Design review of the part built by this model. Coordinates are the model's own, in mm. A direction names the side the tool comes from. Coordinates: 2 decimals unless noted, no trailing zeros. Write each loop counter-clockwise with the first axis right and the second up, starting at its lowest first coordinate (ties: lowest second). Pieces come first, ordered by that corner, then holes. Notation, with made-up numbers: (-5.5, 13.5) -> (35.5, 13.5) arc R19 ccw to (35.5, 45.5) -> close; hole circle Ø7 at (31.5, 74). An arc over 180 degrees is marked (long way). Write item = value, one per line. Start each with the question number.
```python
from build123d import *

# Parameters (mm, degrees)
BOSS_EXTRUDE1_DEPTH      = 90
BOSS_EXTRUDE1_DEPTH_BACK = 10
SKETCH1_W                = 120
SKETCH1_H                = 100
FILLET1_R                = 10
SKETCH2_W                = 80
SKETCH2_H                = 60
CUT_EXTRUDE1_DEPTH       = 127.885775404
SKETCH3_W                = 106.2
SKETCH3_H                = 86.2
SKETCH3_W_2              = 93.8
SKETCH3_H_2              = 73.8
CUT_EXTRUDE2_DEPTH       = 10
BOSS_EXTRUDE3_START      = -20
BOSS_EXTRUDE3_DEPTH      = 80
CUT_EXTRUDE3_START       = -30
SKETCH5_R                = 1.25
CUT_EXTRUDE3_DEPTH       = 60
CUT_EXTRUDE4_DEPTH       = 2.5
SKETCH7_W                = 60
SKETCH7_H                = 4
CUT_EXTRUDE5_DEPTH       = 6
FILLET2_R                = 1.5


with BuildPart() as part:
    # Sketch1 → Boss-Extrude1 (new, two sides: drawn at the far end of the back side and taken through both)
    with BuildSketch(Plane(origin=(0, 0, 0), x_dir=(1, 0, 0), z_dir=(0, 1, 0)).offset(-BOSS_EXTRUDE1_DEPTH_BACK)):
        Rectangle(SKETCH1_W, SKETCH1_H)
    extrude(amount=BOSS_EXTRUDE1_DEPTH + BOSS_EXTRUDE1_DEPTH_BACK)

    # Fillet1
    fillet1_edges = [part.edges().sort_by_distance(p)[0] for p in [
        (-60, 40, -50),
        (60, 40, -50),
        (60, 40, 50),
        (-60, 40, 50),
    ]]
    fillet(fillet1_edges, radius=FILLET1_R)

    # Sketch2 → Cut-Extrude1 (cut, through all)
    with BuildSketch(Plane(origin=(0, 90, 0), x_dir=(1, 0, 0), z_dir=(0, 1, 0))):
        Rectangle(SKETCH2_W, SKETCH2_H)
    extrude(amount=-CUT_EXTRUDE1_DEPTH, mode=Mode.SUBTRACT)

    # Sketch3 → Cut-Extrude2 (cut)
    with BuildSketch(Plane.XZ.offset(10)):
        Rectangle(SKETCH3_W, SKETCH3_H)
        Rectangle(SKETCH3_W_2, SKETCH3_H_2, mode=Mode.SUBTRACT)
    extrude(amount=-CUT_EXTRUDE2_DEPTH, mode=Mode.SUBTRACT)

    # Sketch4 → Boss-Extrude3 (add)
    with BuildSketch(Plane(origin=(60, 0, 0), x_dir=(0, 0, -1), z_dir=(1, 0, 0)).offset(BOSS_EXTRUDE3_START)):
        with BuildLine():
            Line((30, 80), (30, 90))
            ThreePointArc((30, 90), (25, 85), (30, 80))
        make_face()
    extrude(amount=-BOSS_EXTRUDE3_DEPTH)

    # Sketch5 → Cut-Extrude3 (cut)
    with BuildSketch(Plane(origin=(60, 0, 0), x_dir=(0, 0, -1), z_dir=(1, 0, 0)).offset(CUT_EXTRUDE3_START)):
        with BuildLine():
            Line((30, 80), (30, 90))
            ThreePointArc((30, 90), (25, 85), (30, 80))
        make_face()
        with Locations((27.5, 85)):
            Circle(SKETCH5_R, mode=Mode.SUBTRACT)
    extrude(amount=-CUT_EXTRUDE3_DEPTH, mode=Mode.SUBTRACT)

    # Sketch6 → Cut-Extrude4 (cut)
    with BuildSketch(Plane(origin=(0, 90, 0), x_dir=(1, 0, 0), z_dir=(0, 1, 0))):
        with BuildLine():
            Line((-40, -30), (-40, 24))
            Line((-40, 24), (-42, 24))
            Line((-42, 24), (-42, -32))
            Line((-42, -32), (-10.392304845, -32))
            ThreePointArc((-10.392304845, -32), (0, -38), (10.392304845, -32))
            Line((10.392304845, -32), (42, -32))
            Line((42, -32), (42, 24))
            Line((42, 24), (40, 24))
            Line((40, 24), (40, -30))
            Line((40, -30), (-40, -30))
        make_face()
    extrude(amount=-CUT_EXTRUDE4_DEPTH, mode=Mode.SUBTRACT)

    # Sketch7 → Cut-Extrude5 (cut)
    with BuildSketch(Plane(origin=(0, 90, 0), x_dir=(1, 0, 0), z_dir=(0, 1, 0))):
        with Locations((0, 32)):
            Rectangle(SKETCH7_W, SKETCH7_H)
    extrude(amount=-CUT_EXTRUDE5_DEPTH, mode=Mode.SUBTRACT)

    # Fillet2
    fillet2_edges = [part.edges().sort_by_distance(p)[0] for p in [
        (-42, 90, 4),
        (-26.196152423, 90, 32),
        (0, 90, 38),
        (26.196152423, 90, 32),
        (42, 90, 4),
        (0, 84, -34),
        (0, 84, -30),
        (0, 90, -34),
    ]]
    fillet(fillet2_edges, radius=FILLET2_R)


solid = part.part
```
(1) For line 1 (Z direction, x = 37.5, y = 69.5); line 2 (X direction, y = 39, z = 18); line 3 (Y direction, x = 52, z = 32), list the stretches that pass through material, from the lowest coordinate up.
(2) Take a section at A-A, the plane z = 16. State the section outline as (x, y) points.
(3) For pin 1 Ø10 at (x, z) = (-31.5, -4) entering from -Y, flat-tipped, find the tip position at first contact; note if it passes through.
(4) Take a section at D-D, the plane y = 44. State the section outline as (x, z) points.
(5) Take a section at C-C, the plane x = 13.5. State the section outline as (y, z) points, then the cut area to 3 significant figures.
(6) Take a section at B-B, the plane x = 32.5. State the section outline as (y, z) points, then the cut area to 3 significant figures.
(7) For faces 1 (the face through (-35, 85, -25)), 2 (the face through (-1, -5, -43.1)), 3 (the face through (0, 87, -34)), 4 (the face through (-1, 39, 30)), 5 (the face through (-60, 39, 1)), list the 3-axis set-ups (+Z, -Z, +X, -X, +Y, -Y) from which the entire face can be reached by the end or side of a thin tool; tool diameter is ignored.
Report:
q1.line_1 = -50 to -30, 30 to 50
q1.line_2 = -60 to -40, 40 to 60
q1.line_3 = 0 to 90
q2.outline = (-60, -10) -> (-53.1, -10) -> (-53.1, 0) -> (-46.9, 0) -> (-46.9, -10) -> (-40, -10) -> (-40, 87.5) -> (-42, 87.5) -> (-42, 88.5) arc R1.5 ccw to (-43.5, 90) -> (-60, 90) -> close; (40, -10) -> (46.9, -10) -> (46.9, 0) -> (53.1, 0) -> (53.1, -10) -> (60, -10) -> (60, 90) -> (43.5, 90) arc R1.5 ccw to (42, 88.5) -> (42, 87.5) -> (40, 87.5) -> close
q3.pin_1 = through
q4.outline = (-60, -40) arc R10 ccw to (-50, -50) -> (50, -50) arc R10 ccw to (60, -40) -> (60, 40) arc R10 ccw to (50, 50) -> (-50, 50) arc R10 ccw to (-60, 40) -> close; hole (-40, -30) -> (40, -30) -> (40, 30) -> (-40, 30) -> close
q5.outline = (-10, -50) -> (90, -50) -> (90, -35.5) arc R1.5 ccw to (88.5, -34) -> (85.5, -34) arc R1.5 cw to (84, -32.5) -> (84, -31.5) arc R1.5 ccw to (82.5, -30) -> (-10, -30) -> (-10, -36.9) -> (0, -36.9) -> (0, -43.1) -> (-10, -43.1) -> close; (-10, 30) -> (87.5, 30) -> (87.5, 32) -> (88.5, 32) arc R1.5 ccw to (90, 33.5) -> (90, 50) -> (-10, 50) -> (-10, 43.1) -> (0, 43.1) -> (0, 36.9) -> (-10, 36.9) -> close; circle Ø2.5 at (85, -27.5)
q5.area = 3,850 mm2
q6.outline = (-10, -50) -> (90, -50) -> (90, -30) arc R5 ccw to (80, -30) -> (-10, -30) -> (-10, -36.9) -> (0, -36.9) -> (0, -43.1) -> (-10, -43.1) -> close; (-10, 30) -> (87.5, 30) -> (87.5, 32) -> (88.5, 32) arc R1.5 ccw to (90, 33.5) -> (90, 50) -> (-10, 50) -> (-10, 43.1) -> (0, 43.1) -> (0, 36.9) -> (-10, 36.9) -> close
q6.area = 3,910 mm2
q7.face_1 = none
q7.face_2 = -Y
q7.face_3 = +Y
q7.face_4 = +Y, -Y
q7.face_5 = +Z, -Z, -X, +Y, -Y
